For this review, take the finished solid that the model builds, in its own axes (mm). A direction names the side the tool comes from. Coordinates: 2 decimals unless noted, no trailing zeros. Loops run counter-clockwise (first coordinate to the right, second up) from the corner with the lowest first, then second, coordinate; pieces in that order, holes last.
1. Clearance check with flat-ended pins moving along their axes: P1, Ø2, axis at x = 3.5, y = -7, coming from the +Z side; P2, Ø1, axis at x = 1.5, y = 0, coming from the +Z side; P3, Ø2, axis at x = 3, y = -8.5, coming from the -Z side. State where each tip first meets the part, or that it passes through.
2. Take a section at C-C, the plane x = 2.75. State the section outline as (y, z) points, then the cut area to 3 significant figures.
3. Take a section at B-B, the plane z = 5.75. State the section outline as (x, y) points, then the cut area to 3 significant figures.
4. Take a section at D-D, the plane y = -4.5. State the section outline as (x, z) points, then the cut area to 3 significant figures.
5. Mouldability with a two-part tool opening along X and no side actions: class faces 1 (the face through (-5, 1, 5)), 2 (the face through (0.45, 1.01, 1.43)), 3 (the face through (0, 1, -5)) as pulls with the +X half, pulls with the -X half, needs draft (parallel to the pull), parting line crosses it, or undercut.
6. Machinability: for faces 4 (the face through (0, -5, 9.25)), 5 (the face through (0, -10, 11)), which of the approach directions +Z, -Z, +X, -X, +Y, -Y give a long, thin tool a straight path to every point of the face, cutting with its end or side? Answer none if there is none.
7. To check wall thickness, follow probe 1 along X at (y, z) = (1.1, 0); probe 2 along Y at (x, z) = (-2.75, 1.75); probe 3 along Z at (x, y) = (1.25, 0.5). State the ranges of each line that lie inside material, in increasing order.
8. Take a section at A-A, the plane x = 0. State the section outline as (y, z) points, then the cut area to 3 significant figures.
```python
from build123d import *

# Parameters (mm, degrees)
EXTRUDE_1_DEPTH     = 2
SKETCH_2_R          = 1.5
CUT_EXTRUDE_1_DEPTH = 2
EXTRUDE_START       = -12
EXTRUDE_2_DEPTH     = 12


with BuildPart() as part:
    # 草图1 → 凸台-拉伸1 (new body)
    with BuildSketch(Plane(origin=(0, 0, 0), x_dir=(1, 0, 0), z_dir=(0, 1, 0))):
        with BuildLine():
            Line((-5, 0), (-5, -9.25))
            ThreePointArc((-5, -9.25), (0, -14.25), (5, -9.25))
            Line((5, -9.25), (5, 0))
            ThreePointArc((5, 0), (0, 5), (-5, 0))
        make_face()
    extrude(amount=EXTRUDE_1_DEPTH)

    # 草图2 → 切除-拉伸1 (cut)
    with BuildSketch(Plane(origin=(0, 2, 0), x_dir=(1, 0, 0), z_dir=(0, 1, 0))):
        with Locations(Location((0, 0, 0), (0, 0, 270))):
            Circle(SKETCH_2_R)
    extrude(amount=-CUT_EXTRUDE_1_DEPTH, mode=Mode.SUBTRACT)

    # 草图3 → 凸台-拉伸2 (add)
    with BuildSketch(Plane(origin=(0, 2, 0), x_dir=(1, 0, 0), z_dir=(0, 1, 0)).offset(EXTRUDE_START)):
        with BuildLine():
            Line((-5, -9.25), (5, -9.25))
            ThreePointArc((5, -9.25), (0, -14.25), (-5, -9.25))
        make_face()
    extrude(amount=EXTRUDE_2_DEPTH)


solid = part.part
```
Results list:
1. P1: stops at z = 13.58
1. P2: stops at z = 14.15
1. P3: stops at z = 9.25
2. outline: (-10, 9.25) - (0, 9.25) - (0, -4.18) - (2, -4.18) - (2, 13.43) - (-10, 13.43) - close
2. area: 77.0 mm2
3. outline: (-5, 0) - (5, 0) - (5, 2) - (-5, 2) - close
3. area: 20.0 mm2
4. outline: (-5, 9.25) - (5, 9.25) arc R5 ccw to start
4. area: 39.3 mm2
5. face 1: pulls with the -X half
5. face 2: undercut
5. face 3: parting line crosses it
6. face 4: -Z, +X, -X, -Y
6. face 5: +Z, -Z, +X, -X, -Y
7. probe 1: x = -5 to -1.5, 1.5 to 5
7. probe 2: y = 0 to 2
7. probe 3: z = -4.84 to -0.83, 0.83 to 14.09
8. outline: (-10, 9.25) - (0, 9.25) - (0, 1.5) - (2, 1.5) - (2, 14.25) - (-10, 14.25) - close; (0, -5) - (2, -5) - (2, -1.5) - (0, -1.5) - close
8. area: 82.5 mm2
